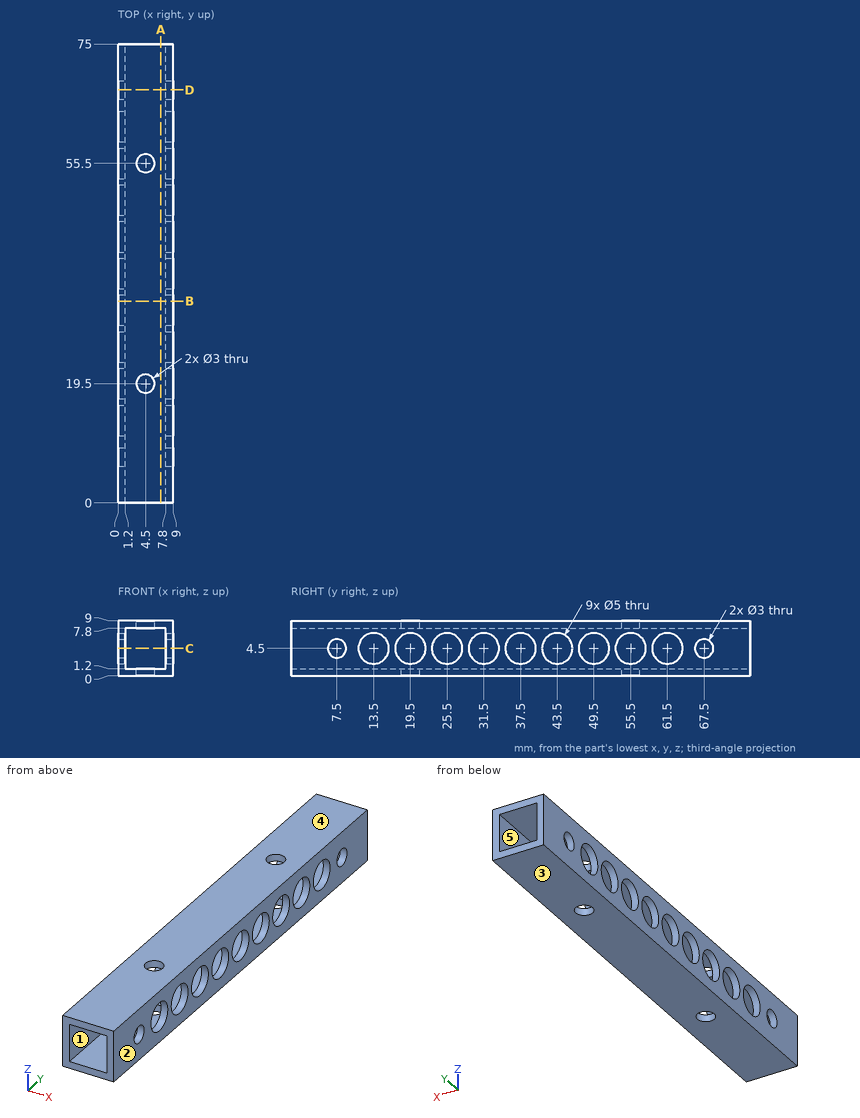
Geometry check sheet. Reference: drawing and pictorial views, mm from the part's lowest x, y, z. A direction names the side the tool comes from. Round coordinates to 2 decimals unless told otherwise and drop trailing zeros. Loops run counter-clockwise (first coordinate to the right, second up) from the corner with the lowest first, then second, coordinate; pieces in that order, holes last. Notation, with made-up numbers: M 24.5,-36 L 41.5,-36 A16 cw 41.5,-13 Z; hole C 89.25,86 d1. An arc over 180 degrees is marked long. Return JSON: item names as keys, results as strings. Group by question number.
(1) Set-up check for the marked faces 4 and 5: record each of +Z, -Z, +X, -X, +Y, -Y from which the full face is reachable in a straight line by a thin tool's end or side.
(2) Section check D-D, the plane y = 67.5. Enter the section's corners in (x, z).
(3) Section check C-C, the plane z = 4.5. Give the number of separate pieces and of enclosed holes in the cut face, and give its area (3 significant figures).
(4) Section check B-B, the plane y = 33. Enter the section's corners in (x, z), and give its area (3 significant figures).
(5) Scan lines: line 1 along Z through (x, y) = (7, 53.5); line 2 along Z through (x, y) = (8.35, 43.5). Record each from-to range of solid material in increasing order. Write a range as [from, to].
(6) Section check A-A, the plane x = 7. Enter the section's corners in (y, z), and give its area (3 significant figures).
(7) Mould release check, pull along Z, two halves, no side actions. Record for the marked faces 1, 2 and 3: pulls with the +Z half, pulls with the -Z half, needs draft (parallel to the pull), parting line crosses it, or undercut.
(8) Go/stop test with a flat-tipped pin: pin 1 (5 mm diameter, centred on x = 5.5, y = 61, fed in from -Z). Record where the tip stops, or that it passes through.
Data:
{
 "1": {"face 4": "+Z, +X, -X, +Y, -Y", "face 5": "+Y, -Y"},
 "2": {"outline": "M 0,0 L 9,0 L 9,3 L 7.8,3 L 7.8,1.2 L 1.2,1.2 L 1.2,3 L 0,3 Z; M 0,6 L 1.2,6 L 1.2,7.8 L 7.8,7.8 L 7.8,6 L 9,6 L 9,9 L 0,9 Z"},
 "3": {"separate pieces": "24", "enclosed holes": "0", "area": "57.6 mm²"},
 "4": {"outline": "M 0,0 L 9,0 L 9,2.5 L 7.8,2.5 L 7.8,1.2 L 1.2,1.2 L 1.2,2.5 L 0,2.5 Z; M 0,6.5 L 1.2,6.5 L 1.2,7.8 L 7.8,7.8 L 7.8,6.5 L 9,6.5 L 9,9 L 0,9 Z", "area": "27.8 mm²"},
 "5": {"line 1": "[0, 1.2], [7.8, 9]", "line 2": "[0, 2], [7, 9]"},
 "6": {"outline": "M 0,0 L 75,0 L 75,1.2 L 0,1.2 Z; M 0,7.8 L 75,7.8 L 75,9 L 0,9 Z", "area": "180 mm²"},
 "7": {"face 1": "undercut", "face 2": "needs draft", "face 3": "pulls with the -Z half"},
 "8": {"pin 1": "z = 0"}
}
